The listing builds one solid part. Answer for the finished solid, in the listing's coordinates (mm). Face numbers are marked on the shaded views. A direction names the side the tool comes from. Round coordinates to 2 decimals unless told otherwise and drop trailing zeros. Write each loop counter-clockwise with the first axis right and the second up, starting at its lowest first coordinate (ties: lowest second). Pieces come first, ordered by that corner, then holes.
(1) A cutting plane is placed at A-A, the plane x = 19.5. Give the vertices of the cut face in (y, z).
(2) For the marked faces 1, 2 and 3, determine the directions among +Z, -Z, +X, -X, +Y, -Y from which every point of the face is accessible in a straight line to the end or side of a thin tool.
(3) Find the intervals of material crossed by probe 1 along X at (y, z) = (-28.6, 5); probe 2 along Z at (x, y) = (-19.5, -29.25); probe 3 along X at (y, z) = (-5, 2.75), in increasing order.
(4) Each of these flat-tipped pins is pushed along its axis until it touches: pin 1 Ø3 at (y, z) = (-0.5, 6) entering from +X; pin 2 Ø1 at (y, z) = (-12.5, 3.5) entering from -X; pin 3 Ø1.5 at (x, z) = (-5.5, 5.5) entering from +Y. Where does it stop, or does it pass through?
(5) A cutting plane is placed at C-C, the plane z = 8.75. Give the vertices of the cut face in (x, y).
(6) A cutting plane is placed at B-B, the plane z = 5. Give the vertices of the cut face in (x, y), and give its area (3 significant figures).
(7) The mould has two halves that part along X. Classify the marked faces 4, 5 and 6: +X half, -X half, draft (parallel to the pull), parting line (faces both ways), or undercut.
(8) A cutting plane is placed at D-D, the plane x = 0. Give the vertices of the cut face in (y, z), and give its area (3 significant figures).
Autodesk Inventor part; units mm, degrees
ref_plane "YZ Plane" through (0, 0, 0) normal (1, 0, 0) x (0, 1, 0)
ref_plane "XZ Plane" through (0, 0, 0) normal (0, 1, 0) x (-1, 0, 0)
ref_plane "XY Plane" through (0, 0, 0) normal (0, 0, 1) x (1, 0, 0)
sketch "Boceto1" plane through (0, 0, 0) normal (0, 0, 1) x (1, 0, 0)
  arc A0 (0, 14) -> (-14, 0) centre (0, 0) ccw
  line L0 (-14, 0) -> (-14, -26.9516)
  line L1 (-14, -26.9516) -> (-25, -26.9516)
  line L2 (-25, -26.9516) -> (-25, -30.9943)
  line L3 (-25, -30.9943) -> (0, -30.9943)
  line L4 (0, -30.9943) -> (0, 14) construction
  arc A1 (0, 7.5) -> (0, -7.5) centre (0, 0) ccw
  arc A2 (14, 0) -> (0, 14) centre (0, 0) ccw
  line L5 (14, 0) -> (14, -26.9516)
  line L6 (14, -26.9516) -> (25, -26.9516)
  line L7 (25, -26.9516) -> (25, -30.9943)
  line L8 (25, -30.9943) -> (0, -30.9943)
  arc A3 (0, -7.5) -> (0, 7.5) centre (0, 0) ccw
  dimension "d2" = 7.5
  dimension "d6" = 50
  dimension "d7" = 28
extrude "Extrusión1" add sketch "Boceto1" along normal blind 10
sketch "Boceto2" plane through (-25, -26.9516, 0) normal (0, 1, 0) x (1, 0, 0)
  line L0 (11, 0) -> (39, 0)
  line L1 (0, -10) -> (50, -10)
  line L2 (11, 0) -> (0, -10)
  line L3 (11, -10) -> (39, -10)
  line L4 (0, 0) -> (50, 0)
  line L5 (11, -10) -> (0, 0)
  line L6 (0, 0) -> (50, -10)
  line L7 (0, -10) -> (50, 0)
  line L8 (25, -5) -> (25, 11.6359)
  circle A0 centre (5.5, -5) radius 2.5
  circle A1 centre (44.5, -5) radius 2.5
  point P0 (25, 0)
  dimension "d3" = 5
extrude "Extrusión2" cut sketch "Boceto2" against normal blind 5 contours A0 L5 L2 | L2 L5 A0 | L5 L2 A0 | L5 A0 L2 | A1
properties part number "sopoetellantas"
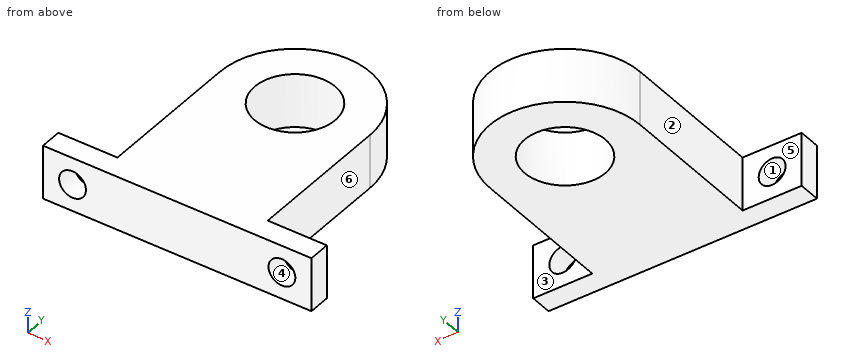
Solutions:
1. outline: (-30.99, 0) - (-26.95, 0) - (-26.95, 2.5) - (-30.99, 2.5) - close; (-30.99, 7.5) - (-26.95, 7.5) - (-26.95, 10) - (-30.99, 10) - close
2. face 1: +Y, -Y
2. face 2: +Z, -Z, -X, +Y
2. face 3: +Z, -Z, +X, +Y
3. probe 1: x = -25 to -22, -17 to 17, 22 to 25
3. probe 2: z = 0 to 2.5, 7.5 to 10
3. probe 3: x = -14 to -5.59, 5.59 to 14
4. pin 1: stops at x = 14
4. pin 2: stops at x = -14
4. pin 3: stops at y = 13.17
5. outline: (-25, -30.99) - (25, -30.99) - (25, -26.95) - (14, -26.95) - (14, 0) arc R14 ccw to (-14, 0) - (-14, -26.95) - (-25, -26.95) - close; hole circle Ø15 at (0, 0)
6. outline: (-25, -30.99) - (-22, -30.99) - (-22, -26.95) - (-25, -26.95) - close; (-17, -30.99) - (17, -30.99) - (17, -26.95) - (14, -26.95) - (14, 0) arc R14 ccw to (-14, 0) - (-14, -26.95) - (-17, -26.95) - close; (22, -30.99) - (25, -30.99) - (25, -26.95) - (22, -26.95) - close; hole circle Ø15 at (0, 0)
6. area: 1,050 mm2
7. face 4: undercut
7. face 5: draft
7. face 6: +X half
8. outline: (-30.99, 0) - (-7.5, 0) - (-7.5, 10) - (-30.99, 10) - close; (7.5, 0) - (14, 0) - (14, 10) - (7.5, 10) - close
8. area: 300 mm2
